Part model, mm, in its own coordinate system. Face numbers are marked on the shaded views. Coordinates: 2 decimals unless noted, no trailing zeros. Order: outer loops, then holes, each group sorted by start corner. A loop starts at its lowest first (then second) coordinate and runs counter-clockwise, first axis right, second up.
1) Wall check: L1, parallel to Z at x = -5.5, y = 9.5 (3 decimals); L2, parallel to X at y = -3.5, z = 46; L3, parallel to Z at x = 31.5, y = 0.25. Give the ranges that are in metal, low to high.
2) Cut at C-C (x = 31.75). List the corners of the cut face in (y, z) (3 decimals), and give its area (3 significant figures).
3) Cut at B-B (x = -31.75). List the corners of the cut face in (y, z), and give its area (3 significant figures).
4) Pin check, flat tips, straight feed: pin 1 Ø2 at (y, z) = (-3, -44.5) entering from +X; pin 2 Ø4 at (x, z) = (31.75, -29.083) entering from -Y; pin 3 Ø6.5 at (x, z) = (0.5, 56) entering from -Y; pin 4 Ø11 at (x, z) = (4, -31.5) entering from -Y. Stop position of each tip, or through.
5) Cut at A-A (x = 17.5). List the corners of the cut face in (y, z) (3 decimals).
6) Mould opens along X. For the marked faces 1, 2 and 3 say: +X half, -X half, draft (parallel to the pull), parting line (faces both ways), or undercut.
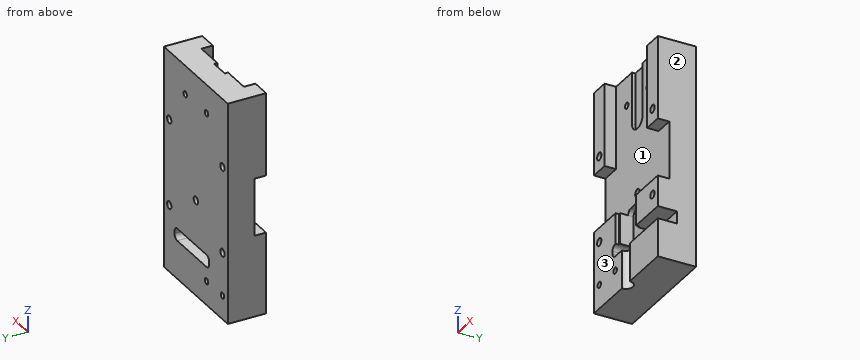
```python
from build123d import *

# Parameters (mm, degrees)
BOSS_EXTRUDE1_DEPTH         = 12.7
BOSS_EXTRUDE1_DEPTH_BACK    = 12.7
SKETCH1_W                   = 76.2
SKETCH1_H                   = 147.066
SKETCH2_R                   = 4.7625
CUT_EXTRUDE1_DEPTH          = 25.4
CUT_EXTRUDE2_DEPTH          = 7.62
CUT_EXTRUDE4_DEPTH          = 84.785452729
CUT_EXTRUDE4_DEPTH_BACK     = 84.785452729
F_1_4_20_TAPPED_HOLE1_D     = 5.1054
F_1_4_20_TAPPED_HOLE1_DEPTH = 19.05
F_1_4_20_TAPPED_HOLE1_TIP   = 1.533816902
SKETCH9_R                   = 2.5527
SKETCH9_R_2                 = 2.0193
CUT_EXTRUDE5_DEPTH          = 87.62489301
CUT_EXTRUDE6_REACH          = 103.385
CUT_EXTRUDE7_DEPTH          = 2.159
SKETCH12_R                  = 2.0193
CUT_EXTRUDE8_DEPTH          = 85.704430162
SKETCH13_W                  = 15.875
SKETCH13_H                  = 8.128
CUT_EXTRUDE9_DEPTH          = 12.7
CUT_EXTRUDE10_DEPTH         = 85.02996052


with BuildPart() as part:
    # Sketch1 → Boss-Extrude1 (new, two sides: drawn at the far end of the back side and taken through both)
    with BuildSketch(Plane(origin=(0, 0, 0), x_dir=(1, 0, 0), z_dir=(0, 1, 0)).offset(-BOSS_EXTRUDE1_DEPTH_BACK)):
        Rectangle(SKETCH1_W, SKETCH1_H)
    extrude(amount=BOSS_EXTRUDE1_DEPTH + BOSS_EXTRUDE1_DEPTH_BACK)

    # Sketch2 → Cut-Extrude1 (cut)
    with BuildSketch(Plane(origin=(0, 0, -73.533), x_dir=(-1, 0, 0), z_dir=(0, 0, -1))):
        with Locations((0, -12.7)):
            Circle(SKETCH2_R)
    extrude(amount=-CUT_EXTRUDE1_DEPTH, mode=Mode.SUBTRACT)

    # Sketch3 → Cut-Extrude2 (cut)
    with BuildSketch(Plane(origin=(0, -12.7, 0), x_dir=(-1, 0, 0), z_dir=(0, -1, 0))):
        with BuildLine():
            Line((-19.05, -83.058), (19.05, -83.058))
            ThreePointArc((19.05, -83.058), (23.540128061, -81.198128061), (25.4, -76.708))
            Line((25.4, -76.708), (25.4, -18.542))
            Line((25.4, -18.542), (44.45, -18.542))
            Line((44.45, -18.542), (44.45, 19.558))
            Line((44.45, 19.558), (-44.45, 19.558))
            Line((-44.45, 19.558), (-44.45, -18.542))
            Line((-44.45, -18.542), (-25.4, -18.542))
            Line((-25.4, -18.542), (-25.4, -76.708))
            ThreePointArc((-25.4, -76.708), (-23.540128061, -81.198128061), (-19.05, -83.058))
        make_face()
    extrude(amount=-CUT_EXTRUDE2_DEPTH, mode=Mode.SUBTRACT)

    # Sketch5 → Cut-Extrude4 (cut, two sides: drawn at the far end of the back side and taken through both)
    with BuildSketch(Plane(origin=(0, 0, 0), x_dir=(1, 0, 0), z_dir=(0, 1, 0)).offset(-CUT_EXTRUDE4_DEPTH_BACK)):
        with BuildLine():
            Line((22.225, 48.133), (-12.7, 48.133))
            ThreePointArc((-12.7, 48.133), (-14.94506403, 47.20306403), (-15.875, 44.958))
            Line((-15.875, 44.958), (-15.875, 43.18))
            ThreePointArc((-15.875, 43.18), (-14.94506403, 40.93493597), (-12.7, 40.005))
            Line((-12.7, 40.005), (22.225, 40.005))
            ThreePointArc((22.225, 40.005), (24.47006403, 40.93493597), (25.4, 43.18))
            Line((25.4, 43.18), (25.4, 44.958))
            ThreePointArc((25.4, 44.958), (24.47006403, 47.20306403), (22.225, 48.133))
        make_face()
    extrude(amount=CUT_EXTRUDE4_DEPTH + CUT_EXTRUDE4_DEPTH_BACK, mode=Mode.SUBTRACT)

    # 1_4-20 Tapped Hole1
    with Locations(Plane(origin=(-11.034450397, 12.7, 14.547513529), x_dir=(-1, 0, 0), z_dir=(0, 1, 0))):
        with Locations((-11.034450397, -24.580513529)):
            Hole(F_1_4_20_TAPPED_HOLE1_D / 2, depth=F_1_4_20_TAPPED_HOLE1_DEPTH)
            with Locations((0, 0, -(F_1_4_20_TAPPED_HOLE1_DEPTH + F_1_4_20_TAPPED_HOLE1_TIP / 2))):  # 118° drill point
                Cone(0, F_1_4_20_TAPPED_HOLE1_D / 2, F_1_4_20_TAPPED_HOLE1_TIP, mode=Mode.SUBTRACT)

    # Sketch9 → Cut-Extrude5 (cut, through all)
    with BuildSketch(Plane(origin=(0, -12.7, 0), x_dir=(-1, 0, 0), z_dir=(0, -1, 0))):
        with Locations(Location((31.75, 29.083, 0), (0, 0, 90))):
            Circle(SKETCH9_R)
        with Locations(Location((31.75, -28.067, 0), (0, 0, 90))):
            Circle(SKETCH9_R)
        with Locations(Location((-31.75, -28.067, 0), (0, 0, 270))):
            Circle(SKETCH9_R)
        with Locations(Location((-31.75, 29.083, 0), (0, 0, 270))):
            Circle(SKETCH9_R)
        with Locations(Location((31.75, 57.658, 0), (0, 0, 90))):
            Circle(SKETCH9_R_2)
        with Locations(Location((12.7, 57.658, 0), (0, 0, 90))):
            Circle(SKETCH9_R_2)
    extrude(amount=-CUT_EXTRUDE5_DEPTH, mode=Mode.SUBTRACT)

    # Sketch10 → Cut-Extrude6 (cut, up to next)
    with BuildSketch(Plane.XY.offset(-19.558), mode=Mode.PRIVATE) as cut_extrude6_sk1:
        with BuildLine():
            Line((-10.939706577, -10.414), (-12.209706577, -10.414))
            Line((-12.209706577, -10.414), (-12.209706577, -14.986))
            Line((-12.209706577, -14.986), (-10.939706577, -14.986))
            ThreePointArc((-10.939706577, -14.986), (0, -23.876), (10.939706577, -14.986))
            Line((10.939706577, -14.986), (12.209706577, -14.986))
            Line((12.209706577, -14.986), (12.209706577, -10.414))
            Line((12.209706577, -10.414), (10.939706577, -10.414))
            Line((10.939706577, -10.414), (10.939706577, -1.524))
            Line((10.939706577, -1.524), (-10.939706577, -1.524))
            Line((-10.939706577, -1.524), (-10.939706577, -10.414))
        make_face()
    cut_extrude6_tool1 = extrude(cut_extrude6_sk1.sketch, amount=-CUT_EXTRUDE6_REACH, mode=Mode.PRIVATE) & part.part
    add(cut_extrude6_tool1.solids().sort_by_distance((0, -11.73366, -19.558))[0], mode=Mode.SUBTRACT)

    # Sketch11 → Cut-Extrude7 (cut)
    with BuildSketch(Plane(origin=(0, -5.08, 0), x_dir=(-1, 0, 0), z_dir=(0, -1, 0))):
        with BuildLine():
            Line((0.00254, -32.893), (-0.00254, -32.893))
            ThreePointArc((-0.00254, -32.893), (-4.490872009, -34.752127991), (-6.35, -39.24046))
            Line((-6.35, -39.24046), (-6.35, -73.533))
            Line((-6.35, -73.533), (6.35, -73.533))
            Line((6.35, -73.533), (6.35, -39.24046))
            ThreePointArc((6.35, -39.24046), (4.490872009, -34.752127991), (0.00254, -32.893))
        make_face()
    extrude(amount=-CUT_EXTRUDE7_DEPTH, mode=Mode.SUBTRACT)

    # Sketch12 → Cut-Extrude8 (cut, through all)
    with BuildSketch(Plane.XZ.offset(5.08)):
        with Locations(Location((12.7, 54.483, 0), (0, 0, 270))):
            Circle(SKETCH12_R)
        with Locations(Location((-12.7, 54.483, 0), (0, 0, 270))):
            Circle(SKETCH12_R)
    extrude(amount=-CUT_EXTRUDE8_DEPTH, mode=Mode.SUBTRACT)

    # Sketch13 → Cut-Extrude9 (cut)
    with BuildSketch(Plane.XZ.offset(12.7)):
        with Locations((30.1625, -44.069)):
            Rectangle(SKETCH13_W, SKETCH13_H)
    extrude(amount=-CUT_EXTRUDE9_DEPTH, mode=Mode.SUBTRACT)

    # Sketch14 → Cut-Extrude10 (cut, through all)
    with BuildSketch(Plane.XZ.offset(1.524)):
        with BuildLine():
            Line((7.764706577, -22.733), (-7.764706577, -22.733))
            ThreePointArc((-7.764706577, -22.733), (-10.939706577, -19.558), (-7.764706577, -16.383))
            Line((-7.764706577, -16.383), (7.764706577, -16.383))
            ThreePointArc((7.764706577, -16.383), (10.939706577, -19.558), (7.764706577, -22.733))
        make_face()
    extrude(amount=CUT_EXTRUDE10_DEPTH, mode=Mode.SUBTRACT)


solid = part.part
```
Geometry check:
1. L1: z = -73.533 to -48.133, -40.005 to 73.533
1. L2: x = -38.1 to -6.35, 6.35 to 38.1
1. L3: z = -73.53 to -31.62, -26.54 to 25.53, 30.61 to 73.53
2. outline: (-12.7, -73.533) - (12.7, -73.533) - (12.7, -31.636) - (-12.7, -31.636) - (-12.7, -40.005) - (0, -40.005) - (0, -48.133) - (-12.7, -48.133) - close; (-12.7, -26.53) - (12.7, -26.53) - (12.7, 25.514) - (-12.7, 25.514) - (-12.7, 18.542) - (-5.08, 18.542) - (-5.08, -19.558) - (-12.7, -19.558) - close; (-12.7, 30.62) - (12.7, 30.62) - (12.7, 73.533) - (-12.7, 73.533) - close
2. area: 3,080 mm2
3. outline: (-12.7, -73.53) - (12.7, -73.53) - (12.7, -59.68) - (-12.7, -59.68) - close; (-12.7, -55.64) - (12.7, -55.64) - (12.7, -31.64) - (-12.7, -31.64) - close; (-12.7, -26.53) - (12.7, -26.53) - (12.7, 25.51) - (-12.7, 25.51) - (-12.7, 18.54) - (-5.08, 18.54) - (-5.08, -19.56) - (-12.7, -19.56) - close; (-12.7, 30.62) - (12.7, 30.62) - (12.7, 73.53) - (-12.7, 73.53) - close
3. area: 3,080 mm2
4. pin 1: stops at x = -15.83
4. pin 2: passes through
4. pin 3: stops at y = -2.92
4. pin 4: stops at y = -1.52
5. outline: (-12.7, -73.533) - (12.7, -73.533) - (12.7, -48.133) - (-12.7, -48.133) - close; (-12.7, -40.005) - (12.7, -40.005) - (12.7, 73.533) - (-5.08, 73.533) - (-5.08, -19.558) - (-12.7, -19.558) - close
6. face 1: undercut
6. face 2: +X half
6. face 3: draft
